Autodesk Inventor part; units mm, degrees
ref_plane "YZ Plane" through (0, 0, 0) normal (1, 0, 0) x (0, 1, 0)
ref_plane "XZ Plane" through (0, 0, 0) normal (0, 1, 0) x (-1, 0, 0)
ref_plane "XY Plane" through (0, 0, 0) normal (0, 0, 1) x (1, 0, 0)
sketch "Sketch1" plane through (0, 0, 0) normal (0, 0, 1) x (1, 0, 0)
  line L0 (3.175, 0) -> (22.225, 0)
  line L1 (25.4, 3.175) -> (25.4, 22.225)
  line L2 (22.225, 25.4) -> (3.175, 25.4)
  line L3 (0, 22.225) -> (0, 3.175)
  arc A0 (3.175, 25.4) -> (0, 22.225) centre (3.175, 22.225) ccw
  arc A1 (0, 3.175) -> (3.175, 0) centre (3.175, 3.175) ccw
  arc A2 (22.225, 0) -> (25.4, 3.175) centre (22.225, 3.175) ccw
  arc A3 (25.4, 22.225) -> (22.225, 25.4) centre (22.225, 22.225) ccw
  line L4 (3.175, 23.4) -> (22.225, 23.4)
  arc A4 (23.4, 22.225) -> (22.225, 23.4) centre (22.225, 22.225) ccw
  line L5 (23.4, 22.225) -> (23.4, 3.175)
  arc A5 (22.225, 2) -> (23.4, 3.175) centre (22.225, 3.175) ccw
  line L6 (22.225, 2) -> (3.175, 2)
  arc A6 (2, 3.175) -> (3.175, 2) centre (3.175, 3.175) ccw
  line L7 (2, 3.175) -> (2, 22.225)
  arc A7 (3.175, 23.4) -> (2, 22.225) centre (3.175, 22.225) ccw
  point P0 (0, 0)
  point P1 (25.4, 0)
  point P2 (0, 25.4)
  dimension "d0" = 25.4
  dimension "d1" = 25.4
  dimension "d2" = 3.175
  dimension "d3" = 2
extrude "Extrusion1" add sketch "Sketch1" along normal blind 1000
sketch "Sketch11" plane through (3.175, 25.4, 1000) normal (0, 1, 0) x (1, 0, 0)
  circle A0 centre (9.525, 500) radius 4.7917
  point P0 (-3.175, 1000)
hole "centerHole" at (12.7, 25.4, 500) direction (0, -1, 0) diameter 11 end through all
sketch "Sketch12" plane through (3.175, 25.4, 1000) normal (0, 1, 0) x (1, 0, 0)
  line L0 (0, 1000) -> (0, 0)
  circle A0 centre (9.525, 927) radius 1.5875
  circle A1 centre (9.525, 777) radius 1.5875
  circle A2 centre (9.525, 627) radius 1.5875
  circle A3 centre (9.525, 500) radius 5.5
  point P0 (-3.175, 1000)
  dimension "d76" = 3.175
  dimension "d80" = 150
  dimension "d140" = 127
hole "longSideHoles" at (12.7, 25.4, 73) at (12.7, 25.4, 223) at (12.7, 25.4, 373) direction (0, -1, 0) diameter 4.5 end through all
sketch "Sketch13" plane through (3.175, 25.4, 1000) normal (0, 1, 0) x (1, 0, 0)
  line L0 (0, 1000) -> (0, 0)
  circle A0 centre (9.525, 68.2) radius 1.5875
  circle A1 centre (9.525, 220.6) radius 1.5875
  circle A2 centre (9.525, 373) radius 1.5875
  circle A3 centre (9.525, 500) radius 5.5
  point P0 (-3.175, 1000)
  dimension "d96" = 152.4
  dimension "d137" = 127
  dimension "d138" = 152.4
hole "shortSideHoles" at (12.7, 25.4, 627) at (12.7, 25.4, 779.4) at (12.7, 25.4, 931.8) direction (0, -1, 0) diameter 4.5 end through all
sketch "Sketch14" plane through (25.4, 22.225, 1000) normal (1, 0, 0) x (0, 0, -1)
  line L0 (1000, -19.05) -> (1000, 0)
  line L1 (0, -19.05) -> (0, 0)
  circle A0 centre (30, -9.525) radius 4.7625
  circle A1 centre (980, -9.525) radius 4.7625
  point P0 (1000, -22.225)
  dimension "d108" = 9.525
  dimension "d109" = 30
  dimension "d110" = 9.525
  dimension "d111" = 20
hole "shackleHole" at (25.4, 12.7, 970) at (25.4, 12.7, 20) direction (-1, 0, 0) diameter 8 end through all
sketch "Sketch15" plane through (3.175, 25.4, 1000) normal (0, 1, 0) x (1, 0, 0)
  circle A0 centre (9.525, 500) radius 5.5
  circle A1 centre (9.525, 560) radius 3.175
  point P0 (-3.175, 1000)
  dimension "d119" = 6.35
  dimension "d120" = 60
hole "collarHole" at (12.7, 25.4, 440) direction (0, -1, 0) diameter 6.6 end through all
sketch "Sketch16" plane through (0, 0, 1000) normal (0, 0, 1) x (1, 0, 0)
  arc A0 (23.4, 22.225) -> (22.225, 23.4) centre (22.225, 22.225) ccw
  line L0 (23.4, 22.225) -> (23.4, 3.175)
  arc A1 (22.225, 2) -> (23.4, 3.175) centre (22.225, 3.175) ccw
  line L1 (22.225, 2) -> (3.175, 2)
  arc A2 (2, 3.175) -> (3.175, 2) centre (3.175, 3.175) ccw
  line L2 (2, 3.175) -> (2, 22.225)
  arc A3 (3.175, 23.4) -> (2, 22.225) centre (3.175, 22.225) ccw
  line L3 (3.175, 23.4) -> (22.225, 23.4)
  line L4 (0, 22.225) -> (0, 3.175)
  arc A4 (0, 3.175) -> (3.175, 0) centre (3.175, 3.175) ccw
  line L5 (3.175, 0) -> (22.225, 0)
  arc A5 (22.225, 0) -> (25.4, 3.175) centre (22.225, 3.175) ccw
  line L6 (25.4, 3.175) -> (25.4, 22.225)
  arc A6 (25.4, 22.225) -> (22.225, 25.4) centre (22.225, 22.225) ccw
  line L7 (22.225, 25.4) -> (3.175, 25.4)
  arc A7 (3.175, 25.4) -> (0, 22.225) centre (3.175, 22.225) ccw
  point P0 (0, 0)
extrude "removeSide" cut sketch "Sketch16" against normal blind 195
equation "\"tube\" = 25.4"
properties part number "2f2al" material "Steel"
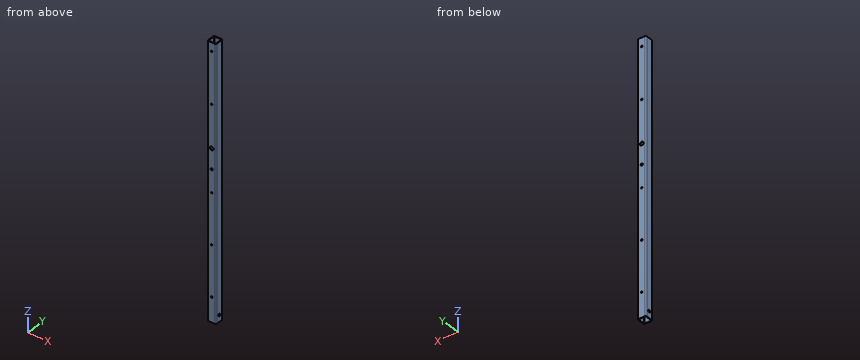
CAD build for the part. Positions are in the model's coordinates, mm. Give positions to 0.01 mm unless a question says otherwise; leave off trailing zeros. Order: outer loops, then holes, each group sorted by start corner. A loop starts at its lowest first (then second) coordinate and runs counter-clockwise, first axis right, second up. Notation, with made-up numbers: (7.25, -40) -> (11.25, -40) arc R15 ccw to (11.25, -22) -> close; hole circle Ø8 at (-16, -36). An arc over 180 degrees is marked (long way). Return JSON: item names as keys, results as strings.
Q1. Saw through at A-A (z = 457.5). Write the cut outline in (x, y) (3 decimals), then the cut area to 3 significant figures.
Working result:
{"outline": "(0, 3.175) arc R3.175 ccw to (3.175, 0) -> (22.225, 0) arc R3.175 ccw to (25.4, 3.175) -> (25.4, 22.225) arc R3.175 ccw to (22.225, 25.4) -> (3.175, 25.4) arc R3.175 ccw to (0, 22.225) -> close; hole (2, 3.175) arc R1.175 ccw to (3.175, 2) -> (22.225, 2) arc R1.175 ccw to (23.4, 3.175) -> (23.4, 22.225) arc R1.175 ccw to (22.225, 23.4) -> (3.175, 23.4) arc R1.175 ccw to (2, 22.225) -> close", "area": "180 mm²"}
Q2. Flat gauge pin, fed straight in: pin 1 (6 mm diameter, centred on x = 22.5, y = 22.5, fed in from -Z). Where does the tip first touch, or does it go through?
Working result:
{"pin 1": "z = 0"}
Q3. Drill centre lines: line 1 (X direction, y = 7, z = 101); line 2 (X direction, y = 0.65, z = 223). Where is each one in solid material? Low to high.
Working result:
{"line 1": "0 to 2, 23.4 to 25.4", "line 2": "1.25 to 10.45, 14.95 to 24.15"}
